Design review of the part built by this model. Coordinates are the model's own, in mm. A direction names the side the tool comes from. Round coordinates to 2 decimals unless told otherwise and drop trailing zeros. Loops run counter-clockwise (first coordinate to the right, second up) from the corner with the lowest first, then second, coordinate; pieces in that order, holes last. Notation, with made-up numbers: M 39,-29.5 L 60,-29.5 A34 cw 60,6.5 Z; hole C 1.5,-15.75 d11. An arc over 180 degrees is marked long. Use a Markdown table: item, result.
Autodesk Inventor part; units mm, degrees
ref_plane "YZ Plane" through (0, 0, 0) normal (1, 0, 0) x (0, 1, 0)
ref_plane "XZ Plane" through (0, 0, 0) normal (0, 1, 0) x (-1, 0, 0)
ref_plane "XY Plane" through (0, 0, 0) normal (0, 0, 1) x (1, 0, 0)
sketch "Skizze1" plane through (0, 0, 0) normal (0, 0, 1) x (1, 0, 0)
  circle A0 centre (0, 0) radius 5
  circle A1 centre (0, 0) radius 4
  dimension "d0" = 8
  dimension "d1" = 10
extrude "Extrusion1" add sketch "Skizze1" along normal blind 12
sketch "Skizze2" plane through (0, 0, 12) normal (0, 0, 1) x (1, 0, 0)
  circle A0 centre (0, 0) radius 5
  line L0 (-2.8868, 5) -> (2.8868, 5)
  line L1 (2.8868, 5) -> (5.7735, 0)
  line L2 (5.7735, 0) -> (2.8868, -5)
  line L3 (2.8868, -5) -> (-2.8868, -5)
  line L4 (-2.8868, -5) -> (-5.7735, 0)
  line L5 (-5.7735, 0) -> (-2.8868, 5)
extrude "Extrusion2" add sketch "Skizze2" against normal blind 3 contours A0 L1 L2 | A0 L0 L1 | L2 L3 A0 | A0 L5 L0 | L3 L4 A0 | A0 L4 L5
sketch "Skizze3" plane through (5.7735, 0, 12) normal (0.8660254, -0.5, 0) x (0, 0, -1)
  line L0 (0, 0) -> (0, -5.7735)
  line L1 (0, -2.8868) -> (12, -2.8868) construction
  point P0 (9.5, -2.8868)
  dimension "d6" = 2.5
hole "Bohrung1" at (4.3301, -2.5, 2.5) direction (-0.8660254, 0.5, 0) diameter 3 depth 4 tip angle 118
properties part number "messingnut" material "Messing, weicher Gelbton"
1. Take a section at D-D on y = -1.75. Count the separate pieces of the cut face and the enclosed holes in it, and give its area (3 significant figures).
Check values:
| item | result |
|---|---|
| separate pieces | 3 |
| enclosed holes | 0 |
| area | 23.6 mm² |
2. Take a section at C-C on z = 6. Give the boundary of the cut face in (x, y), and give its area (3 significant figures).
Check values:
| item | result |
|---|---|
| outline | C 0,0 d10; hole C 0,0 d8 |
| area | 28.3 mm² |
3. Machinability: for faces 4 (the face through (5.2, 0, 9)), 5 (the face through (2.6, -4.5, 9)), 6 (the face through (-4, 3, 4)), which of the approach directions +Z, -Z, +X, -X, +Y, -Y give a long, thin tool a straight path to every point of the face, cutting with its end or side? Answer none if there is none.
Check values:
| item | result |
|---|---|
| face 4 | -Z, +X |
| face 5 | -Z, +X, -Y |
| face 6 | -Z |
4. The part is to be moulded in two halves that separate along Z. For faces 1 (the face through (4.5, -0.9, 2.8)), 2 (the face through (-2.7, 4.5, 9)), 3 (the face through (0, 5, 11)), say which applies: pulls with the +Z half, pulls with the -Z half, needs draft (parallel to the pull), parting line crosses it, or undercut.
Check values:
| item | result |
|---|---|
| face 1 | undercut |
| face 2 | pulls with the -Z half |
| face 3 | needs draft |
5. Insertion check: pin 1 (1.3 mm diameter, centred on x = 2, y = 3.5, fed in from -Z); pin 2 (1.5 mm diameter, centred on y = 2.5, z = 10, fed in from -X); pin 3 (4 mm diameter, centred on y = -1.5, z = 5.5, fed in from +X); pin 4 (1 mm diameter, centred on x = -4, z = 9.5, fed in from +Y). Each pin has a flat end and moves straight along its axis. Give the tip position at first contact, or say it passes through.
Check values:
| item | result |
|---|---|
| pin 1 | stops at z = 0 |
| pin 2 | stops at x = -4.76 |
| pin 3 | stops at x = 5 |
| pin 4 | stops at y = 3.94 |
6. Wall thickness on line 1 along Y through (x, z) = (0, 4.75); line 2 along Z through (x, y) = (2.75, -4.25); line 3 along Y through (x, z) = (2.25, 5): over which ranges is each line inside the solid? List them lowest first. Write a range as from..to.
Check values:
| item | result |
|---|---|
| line 1 | y = -5..-4, 4..5 |
| line 2 | z = 9..12 |
| line 3 | y = -4.47..-3.31, 3.31..4.47 |
7. Take a section at A-A on y = 0.75. Give the boundary of the cut face in (x, z).
Check values:
| item | result |
|---|---|
| outline | M -5.34,9 L -4.94,9 L -4.94,0 L -3.93,0 L -3.93,12 L -5.34,12 Z; M 3.93,0 L 4.94,0 L 4.94,9 L 5.34,9 L 5.34,12 L 3.93,12 Z |
8. Take a section at B-B on x = -3.25. Give the boundary of the cut face in (y, z).
Check values:
| item | result |
|---|---|
| outline | M -4.37,9 L -3.8,9 L -3.8,0 L -2.33,0 L -2.33,12 L -4.37,12 Z; M 2.33,0 L 3.8,0 L 3.8,9 L 4.37,9 L 4.37,12 L 2.33,12 Z |
